Design review of the part built by this model. Coordinates are the model's own, in mm. Face numbers are marked on the shaded views. A direction names the side the tool comes from. Round coordinates to 2 decimals unless told otherwise and drop trailing zeros. Loops run counter-clockwise (first coordinate to the right, second up) from the corner with the lowest first, then second, coordinate; pieces in that order, holes last. Notation, with made-up numbers: M 57,-9.5 L 88,-9.5 A14 cw 88,10.5 Z; hole C 6.25,0 d7. An arc over 180 degrees is marked long. One line per item, written item: value. Start each with the question number.
Item 1: We need section B-B (z = -28.5). Write out the cut boundary in (x, y).
Item 2: Clearance check with flat-ended pins moving along their axes: pin 1 (1.5 mm diameter, centred on x = 16, y = -23.5, fed in from -Z); pin 2 (13 mm diameter, centred on y = -47.7, z = -27.85, fed in from +X); pin 3 (10 mm diameter, centred on x = 17.5, z = -20.5, fed in from -Y); pin 4 (3 mm diameter, centred on y = -46.5, z = -44, fed in from +X). State where each tip first meets the part, or that it passes through.
Item 3: We need section C-C (x = 21.5). Write out the cut boundary in (y, z), then the cut area to 3 significant figures.
Item 4: For the marked faces 1, 2, 3, 4 and 5, list the 3-axis set-ups (+Z, -Z, +X, -X, +Y, -Y) from which the entire face can be reached by the end or side of a thin tool; tool diameter is ignored.
Item 5: We need section D-D (y = -12). Write out the cut boundary in (x, z), then the cut area to 3 significant figures.
Item 6: We need section A-A (y = -47). Write out the cut boundary in (x, z).
Item 7: For line 1 along Z through (x, y) = (13.5, -47.5); line 2 along X through (y, z) = (-20.5, -42); line 3 along Z through (x, y) = (16, -42.5), list the stretches that pass through material, from the lowest coordinate up.
Item 8: Mouldability with a two-part tool opening along Y and no side actions: class the marked faces 6, 7 and 8 as released by +Y, released by -Y, zero draft, split by the parting line, or undercut.
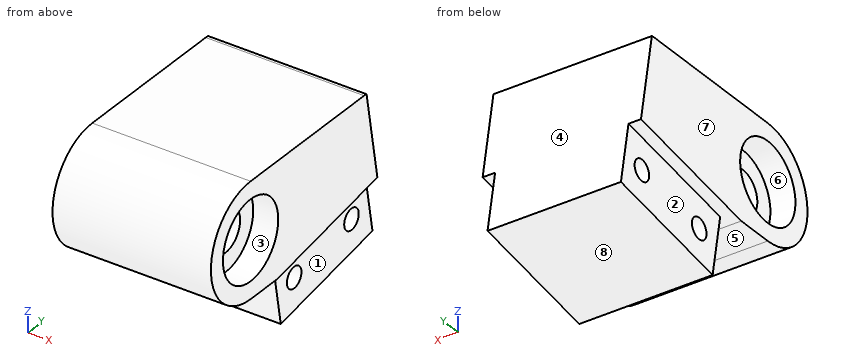
from build123d import *

# Parameters (mm, degrees)
SKETCH1_R           = 5
BOSS_EXTRUDE1_DEPTH = 38
SKETCH2_R           = 9.5
CUT_EXTRUDE1_DEPTH  = 6
SKETCH3_W           = 38
SKETCH3_H           = 38
SKETCH3_W_2         = 32
SKETCH3_H_2         = 32
CUT_EXTRUDE2_DEPTH  = 15
SKETCH4_W           = 38
SKETCH4_H           = 3
CUT_EXTRUDE3_DEPTH  = 31.815956095
SKETCH6_R           = 2.5
CUT_EXTRUDE4_DEPTH  = 36


with BuildPart() as part:
    # Sketch1 → Boss-Extrude1 (new body)
    with BuildSketch(Plane(origin=(0, 0, 0), x_dir=(0, 0, -1), z_dir=(1, 0, 0))):
        with BuildLine():
            Line((18.027765774, -4.140855059), (49.663434225, 1.437366842))
            Line((49.663434225, 1.437366842), (56.262064976, -35.985327773))
            Line((56.262064976, -35.985327773), (41.489948681, -38.590050438))
            Line((41.489948681, -38.590050438), (41.489948681, -47.702008996))
            ThreePointArc((41.489948681, -47.702008996), (27.850151899, -61.341805778), (14.210355117, -47.702008996))
            Line((14.210355117, -47.702008996), (14.210355117, -8.690267924))
            ThreePointArc((14.210355117, -8.690267924), (15.291135012, -5.720849566), (18.027765774, -4.140855059))
        make_face()
        with Locations((27.850151899, -47.702008996)):
            Circle(SKETCH1_R, mode=Mode.SUBTRACT)
    extrude(amount=BOSS_EXTRUDE1_DEPTH)

    # Sketch2 → Cut-Extrude1 (cut)
    with BuildSketch(Plane(origin=(38, 0, 0), x_dir=(0, 0, -1), z_dir=(1, 0, 0))):
        with Locations((27.850151899, -47.702008996)):
            Circle(SKETCH2_R)
    cut_extrude1 = extrude(amount=-CUT_EXTRUDE1_DEPTH, mode=Mode.SUBTRACT)

    # Mirror1: Cut-Extrude1 across plane
    add(cut_extrude1.mirror(Plane(origin=(19, 0, 0), x_dir=(0, 0, 1), z_dir=(1, 0, 0))), mode=Mode.SUBTRACT)

    # Sketch3 → Cut-Extrude2 (cut)
    with BuildSketch(Plane(origin=(0, 8.536289359, -48.411702651), x_dir=(-1, 0, 0), z_dir=(0, 0.173648178, -0.984807753))):
        with Locations((-19, -26.20843484)):
            Rectangle(SKETCH3_W, SKETCH3_H)
        with Locations((-19, -26.20843484)):
            Rectangle(SKETCH3_W_2, SKETCH3_H_2, mode=Mode.SUBTRACT)
    extrude(amount=-CUT_EXTRUDE2_DEPTH, mode=Mode.SUBTRACT)

    # Sketch4 → Cut-Extrude3 (cut, through all)
    with BuildSketch(Plane(origin=(0, 5.931566694, -33.639586356), x_dir=(-1, 0, 0), z_dir=(0, 0.173648178, -0.984807753))):
        with Locations((-19, -8.70843484)):
            Rectangle(SKETCH4_W, SKETCH4_H)
    extrude(amount=-CUT_EXTRUDE3_DEPTH, mode=Mode.SUBTRACT)

    # Sketch6 → Cut-Extrude4 (cut, through all)
    with BuildSketch(Plane(origin=(35, 0, 0), x_dir=(0, 0, -1), z_dir=(1, 0, 0))):
        with Locations((43.840209676, -8.728264268)):
            Circle(SKETCH6_R)
        with Locations((47.31317323, -28.424419328)):
            Circle(SKETCH6_R)
    extrude(amount=-CUT_EXTRUDE4_DEPTH, mode=Mode.SUBTRACT)


solid = part.part
A:
1. outline: M 0,-61.33 L 38,-61.33 L 38,-57.18 L 32,-57.18 L 32,-52.66 L 6,-52.66 L 6,-57.18 L 0,-57.18 Z; M 0,-38.22 L 6,-38.22 L 6,-42.74 L 32,-42.74 L 32,-38.22 L 38,-38.22 L 38,-5.34 L 0,-5.34 Z
2. pin 1: z = -54.19
2. pin 2: x = 32
2. pin 3: y = -61.14
2. pin 4: through
3. outline: M -47.7,-41.49 L -38.59,-41.49 L -35.64,-40.97 L -33.03,-55.74 L -1.52,-50.18 L -7.85,-14.29 A4.62 ccw -8.69,-14.21 L -47.7,-14.21 A13.64 ccw Z; hole C -47.7,-27.85 d10; hole C -28.42,-47.31 d5; hole C -8.73,-43.84 d5
3. area: 1,700 mm2
4. face 1: -Z, +X, +Y
4. face 2: -Z, -X, +Y
4. face 3: +X
4. face 4: +Z, +X, -X, +Y
4. face 5: -Z, +X, -X, -Y
5. outline: M 0,-36.8 L 3,-36.8 L 3,-52.03 L 35,-52.03 L 35,-36.8 L 38,-36.8 L 38,-14.21 L 0,-14.21 Z
5. area: 1,350 mm2
6. outline: M 0,-41.49 L 38,-41.49 L 38,-37.32 L 32,-37.32 L 32,-32.8 L 6,-32.8 L 6,-37.32 L 0,-37.32 Z; M 0,-18.38 L 6,-18.38 L 6,-22.9 L 32,-22.9 L 32,-18.38 L 38,-18.38 L 38,-14.21 L 0,-14.21 Z
7. line 1: -41.49 to -32.85, -22.85 to -14.21
7. line 2: 3 to 35
7. line 3: -41.49 to -14.21
8. face 6: undercut
8. face 7: zero draft
8. face 8: released by +Y
